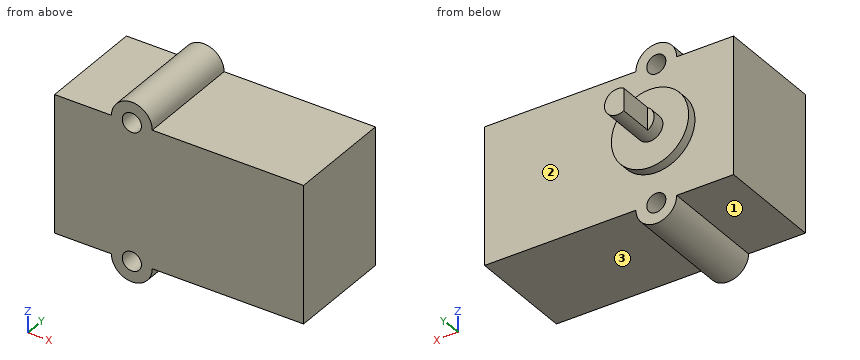
```python
from build123d import *

# Parameters (mm, degrees)
SKETCH1_R           = 2.225
BOSS_EXTRUDE1_DEPTH = 25
SKETCH2_R           = 9
BOSS_EXTRUDE2_DEPTH = 2.2
SKETCH3_R           = 3
BOSS_EXTRUDE3_DEPTH = 11.35
SKETCH4_W           = 1.5
SKETCH4_H           = 6
CUT_EXTRUDE1_DEPTH  = 8.3


with BuildPart() as part:
    # Sketch1 → Boss-Extrude1 (new body)
    with BuildSketch(Plane(origin=(0, 0, 0), x_dir=(1, 0, 0), z_dir=(0, 1, 0))):
        with BuildLine():
            Line((-5.75, -16), (-19, -16))
            Line((-19, -16), (-19, 16))
            Line((-19, 16), (-5.75, 16))
            ThreePointArc((-5.75, 16), (-1, 20.75), (3.75, 16))
            Line((3.75, 16), (39, 16))
            Line((39, 16), (39, -16))
            Line((39, -16), (3.75, -16))
            ThreePointArc((3.75, -16), (-1, -20.75), (-5.75, -16))
        make_face()
        with Locations(Location((-1, -16, 0), (0, 0, 270))):
            Circle(SKETCH1_R, mode=Mode.SUBTRACT)
        with Locations(Location((-1, 16, 0), (0, 0, 90))):
            Circle(SKETCH1_R, mode=Mode.SUBTRACT)
    extrude(amount=BOSS_EXTRUDE1_DEPTH)

    # Sketch2 → Boss-Extrude2 (add)
    with BuildSketch(Plane(origin=(0, 25, 0), x_dir=(1, 0, 0), z_dir=(0, 1, 0))):
        with Locations(Location((-1, 0, 0), (0, 0, 270))):
            Circle(SKETCH2_R)
    extrude(amount=BOSS_EXTRUDE2_DEPTH)

    # Sketch3 → Boss-Extrude3 (add)
    with BuildSketch(Plane(origin=(0, 27.2, 0), x_dir=(1, 0, 0), z_dir=(0, 1, 0))):
        with Locations(Location((-1, 0, 0), (0, 0, 270))):
            Circle(SKETCH3_R)
    extrude(amount=BOSS_EXTRUDE3_DEPTH)

    # Sketch4 → Cut-Extrude1 (cut)
    with BuildSketch(Plane(origin=(0, 38.55, 0), x_dir=(1, 0, 0), z_dir=(0, 1, 0))):
        with Locations((-3.25, 0)):
            Rectangle(SKETCH4_W, SKETCH4_H)
    extrude(amount=-CUT_EXTRUDE1_DEPTH, mode=Mode.SUBTRACT)


solid = part.part
```
The listing builds one solid part. Answer for the finished solid, in the listing's coordinates (mm). Face numbers are marked on the shaded views. A direction names the side the tool comes from. Give positions to 0.01 mm unless a question says otherwise; leave off trailing zeros. Order: outer loops, then holes, each group sorted by start corner. A loop starts at its lowest first (then second) coordinate and runs counter-clockwise, first axis right, second up.
Item 1: Find the intervals of material crossed by probe 1 along Z at (x, y) = (-13.5, 8); probe 2 along Y at (x, z) = (-13, 10.5); probe 3 along Y at (x, z) = (-0.5, 8), in increasing order.
From the geometry:
probe 1: z = -16 to 16
probe 2: y = 0 to 25
probe 3: y = 0 to 27.2
Item 2: The part is cut by section A-A, the plane x = -1. Give the vertices of the cut face in (y, z) (3 decimals), and give its area (3 significant figures).
From the geometry:
outline: (0, -20.75) - (25, -20.75) - (25, -18.225) - (0, -18.225) - close; (0, -13.775) - (25, -13.775) - (25, -9) - (27.2, -9) - (27.2, -3) - (38.55, -3) - (38.55, 3) - (27.2, 3) - (27.2, 9) - (25, 9) - (25, 13.775) - (0, 13.775) - close; (0, 18.225) - (25, 18.225) - (25, 20.75) - (0, 20.75) - close
area: 923 mm2
Item 3: The part is cut by section C-C, the plane z = 0. Give the vertices of the cut face in (x, y), and give its area (3 significant figures).
From the geometry:
outline: (-19, 0) - (39, 0) - (39, 25) - (8, 25) - (8, 27.2) - (2, 27.2) - (2, 38.55) - (-2.5, 38.55) - (-2.5, 30.25) - (-4, 30.25) - (-4, 27.2) - (-10, 27.2) - (-10, 25) - (-19, 25) - close
area: 1,550 mm2
Item 4: The part is cut by section B-B, the plane y = 16. Give the vertices of the cut face in (x, z) (3 decimals), and give its area (3 significant figures).
From the geometry:
outline: (-19, -16) - (-5.75, -16) arc R4.75 ccw to (3.75, -16) - (39, -16) - (39, 16) - (3.75, 16) arc R4.75 ccw to (-5.75, 16) - (-19, 16) - close; hole circle Ø4.45 at (-1, -16); hole circle Ø4.45 at (-1, 16)
area: 1,900 mm2
Item 5: Given pin 1 Ø4 at (y, z) = (36, 1) entering from -X; pin 2 Ø14.5 at (x, y) = (-11.5, 18) entering from +Z; pin 3 Ø20 at (x, y) = (16, 9) entering from +Z; pin 4 Ø9 at (x, z) = (0, -3.5) entering from +Y, each flat-ended and moving along its own axis, determine where each tip first touches the part or whether it passes through.
From the geometry:
pin 1: stops at x = -2.5
pin 2: stops at z = 19.46
pin 3: stops at z = 16
pin 4: stops at y = 38.55
Item 6: Which of the six approach directions +Z, -Z, +X, -X, +Y, -Y give full straight-line access (tool end or side, diameter ignored) to the marked faces 1, 2 and 3?
From the geometry:
face 1: -Z, -X, +Y, -Y
face 2: +Y
face 3: -Z, +X, +Y, -Y
Item 7: The part is cut by section D-D, the plane x = 5. Give the vertices of the cut face in (y, z), and give its area (3 significant figures).
From the geometry:
outline: (0, -16) - (25, -16) - (25, -6.71) - (27.2, -6.71) - (27.2, 6.71) - (25, 6.71) - (25, 16) - (0, 16) - close
area: 830 mm2
